The figure shows three views and two pictorial views of one solid part (mm, origin at its lowest corner). Answer the questions. A direction names the side the tool comes from. Give positions to 0.01 mm unless a question says otherwise; leave off trailing zeros. Loops run counter-clockwise (first coordinate to the right, second up) from the corner with the lowest first, then second, coordinate; pieces in that order, holes last. Notation, with made-up numbers: (13, 63) - (17, 63) arc R29 ccw to (17, 87) - close; hole circle Ø6 at (25.25, -0.75). An arc over 180 degrees is marked (long way). Use CSV: the item, a comma, the result in double quotes.
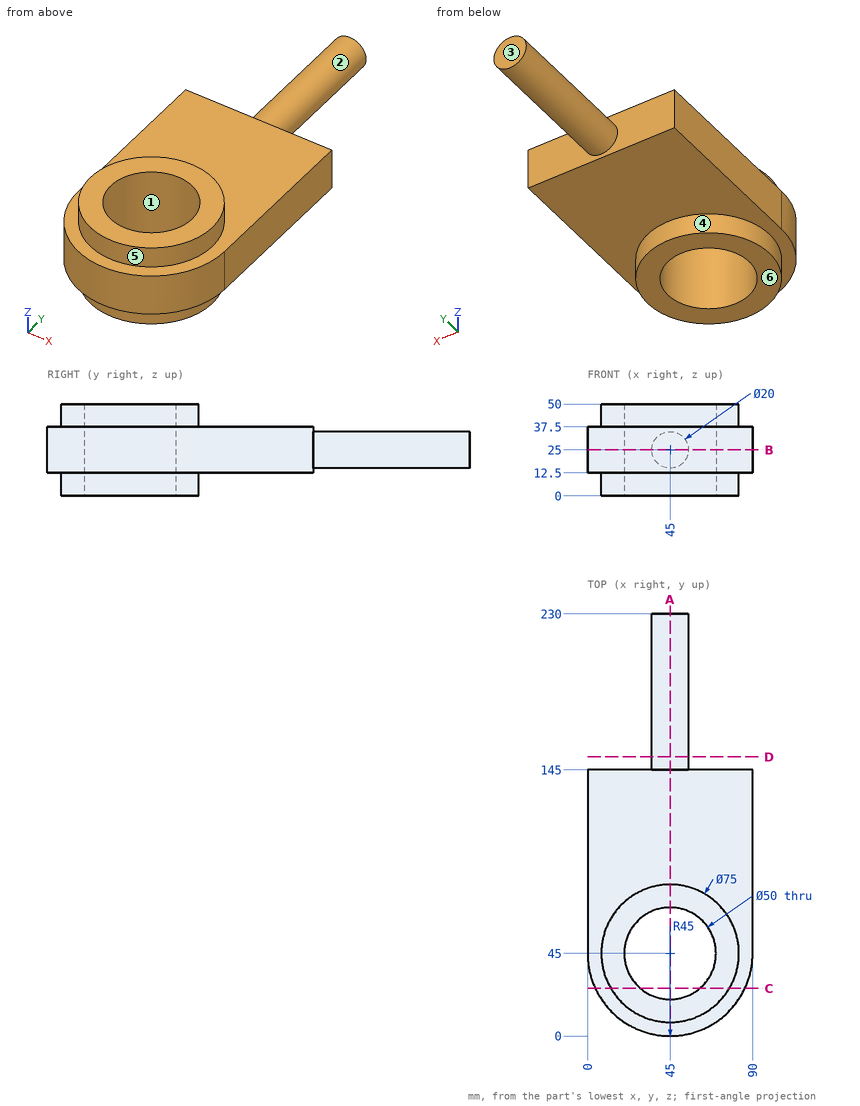
Item 1: For the marked faces 4, 5 and 6, determine the directions among +Z, -Z, +X, -X, +Y, -Y from which every point of the face is accessible in a straight line to the end or side of a thin tool.
Determined:
face 4,"-Z"
face 5,"+Z"
face 6,"-Z, +X, -X, +Y, -Y"
Item 2: A cutting plane is placed at A-A on x = 45. Determine the outline of the cut face in (y, z).
Determined:
outline,"(0, 12.5) - (7.5, 12.5) - (7.5, 0) - (20, 0) - (20, 50) - (7.5, 50) - (7.5, 37.5) - (0, 37.5) - close; (70, 0) - (82.5, 0) - (82.5, 12.5) - (145, 12.5) - (145, 15) - (230, 15) - (230, 35) - (145, 35) - (145, 37.5) - (82.5, 37.5) - (82.5, 50) - (70, 50) - close"
Item 3: A cutting plane is placed at B-B on z = 25. Determine the outline of the cut face in (x, y), and give its area (3 significant figures).
Determined:
outline,"(0, 45) arc R45 ccw to (90, 45) - (90, 145) - (55, 145) - (55, 230) - (35, 230) - (35, 145) - (0, 145) - close; hole circle Ø50 at (45, 45)"
area,"11,900 mm²"
Item 4: The mould has two halves that part along X. Classify the marked faces 1, 2 and 3: pulls with the +X half, pulls with the -X half, needs draft (parallel to the pull), parting line crosses it, or undercut.
Determined:
face 1,"undercut"
face 2,"parting line crosses it"
face 3,"needs draft"
Item 5: A cutting plane is placed at C-C on y = 26. Determine the outline of the cut face in (x, z).
Determined:
outline,"(4.21, 12.5) - (12.67, 12.5) - (12.67, 0) - (28.75, 0) - (28.75, 50) - (12.67, 50) - (12.67, 37.5) - (4.21, 37.5) - close; (61.25, 0) - (77.33, 0) - (77.33, 12.5) - (85.79, 12.5) - (85.79, 37.5) - (77.33, 37.5) - (77.33, 50) - (61.25, 50) - close"
Item 6: Given P1, Ø5, axis at y = 95.5, z = 9.5, coming from the +X side; P2, Ø12, axis at x = 60, y = 205, coming from the +Z side; P3, Ø8, axis at x = 15.5, y = 123.5, coming from the +Z side; P4, Ø1.5, axis at x = 17.5, z = 14.5, coming from the -Y side, each flat-ended and moving along its own axis, determine where each tip first touches the part or whether it passes through.
Determined:
P1,"passes through"
P2,"stops at z = 29.36"
P3,"stops at z = 37.5"
P4,"stops at y = 8.81"
Item 7: Find the intervals of material crossed by line 1 (Y direction, x = 45, z = 30); line 2 (Z direction, x = 67, y = 123); line 3 (Y direction, x = 26, z = 20), in increasing order.
Determined:
line 1,"y = 0 to 20, 70 to 230"
line 2,"z = 12.5 to 37.5"
line 3,"y = 4.21 to 28.75, 61.25 to 145"
Item 8: A cutting plane is placed at D-D on y = 152. Determine the outline of the cut face in (x, z).
Determined:
outline,"circle Ø20 at (45, 25)"
